The model under review builds one solid part; all positions refer to its coordinate system, in mm. A direction names the side the tool comes from. Coordinates: 2 decimals unless noted, no trailing zeros. Write each loop counter-clockwise with the first axis right and the second up, starting at its lowest first coordinate (ties: lowest second). Pieces come first, ordered by that corner, then holes. Notation, with made-up numbers: M 14,-9.5 L 37,-9.5 A12 ccw 37,2.5 Z; hole C 61,84 d2. An arc over 180 degrees is marked long. Answer as a JSON object with one key per item and string values.
Autodesk Fusion 360 part; units mm, degrees
sketch "Sketch1" plane through (0, 0, 0) normal (0, 0, 1) x (1, 0, 0)
  circle A0 centre (0, 0) radius 11
  circle A1 centre (0, 0) radius 12.5
  circle A2 centre (0, 0) radius 14.5
  line L0 (0, 0) -> (0, 14.5)
  line L1 (0, 0) -> (14.5, 0)
  line L2 (0, 0) -> (-14.5, 0)
  line L3 (0, 0) -> (0, -14.5)
  circle A3 centre (0, 14.5) radius 3.5
  circle A4 centre (14.5, 0) radius 3.5
  circle A5 centre (0, -14.5) radius 3.5
  circle A6 centre (-14.5, 0) radius 3.5
  circle A7 centre (-14.5, 0) radius 1.5
  circle A8 centre (0, 14.5) radius 1.5
  circle A9 centre (14.5, 0) radius 1.5
  circle A10 centre (0, -14.5) radius 1.5
  dimension "d1" = 22
  dimension "d2" = 25
  dimension "d3" = 29
  dimension "d4" = 7
  dimension "d5" = 3
  dimension "d6" = 3
  dimension "d7" = 3
  dimension "d8" = 3
extrude "Extrude1" add sketch "Sketch1" along normal blind 1 contours A0 A1 A4 A5 | A1 L1 A4 | A0 A1 A3 A4 | A1 L1 A4 | A1 L0 A3 | A0 A1 A3 A6 | A1 L0 A3 | A0 A1 A5 A6 | A1 L3 A5 | A1 L3 A5 | A1 A2 L1 A4 A9 | A1 A2 L1 A4 A9 | A1 A2 A3 A4 | A1 A2 A4 A5 | A1 L2 A6 | A1 L2 A6 | A1 A2 L0 A3 A8 | A1 A2 L0 A3 A8 | A1 A2 A3 A6 | A1 A2 L3 A5 A10 | A1 A2 L3 A5 A10 | A1 A2 A5 A6 | A2 A4 A9 | A1 A2 L2 A6 A7 | A1 A2 L2 A6 A7 | A2 A3 A8 | A2 A5 A10 | A2 A6 A7
sketch "Sketch2" plane through (0, 0, 1) normal (0, 0, 1) x (1, 0, 0)
  circle A0 centre (0, -14.5) radius 1.5
  circle A1 centre (14.5, 0) radius 1.5
  circle A2 centre (-14.5, 0) radius 1.5
  circle A3 centre (0, 14.5) radius 1.5
  circle A4 centre (0, 0) radius 11
  arc A5 (-3.4744, 14.0776) -> (-14.0776, 3.4744) centre (0, 0) ccw
  arc A6 (-14.0776, 3.4744) -> (-14.0776, -3.4744) centre (-14.5, 0) ccw
  arc A7 (-14.0776, -3.4744) -> (-3.4744, -14.0776) centre (0, 0) ccw
  arc A8 (-3.4744, -14.0776) -> (3.4744, -14.0776) centre (0, -14.5) ccw
  arc A9 (3.4744, -14.0776) -> (14.0776, -3.4744) centre (0, 0) ccw
  arc A10 (14.0776, -3.4744) -> (14.0776, 3.4744) centre (14.5, 0) ccw
  arc A11 (14.0776, 3.4744) -> (3.4744, 14.0776) centre (0, 0) ccw
  arc A12 (3.4744, 14.0776) -> (-3.4744, 14.0776) centre (0, 14.5) ccw
  circle A13 centre (0, 0) radius 11
  circle A14 centre (0, 0) radius 12.375
  circle A15 centre (0, 0) radius 14.5
  circle A16 centre (0, 14.5) radius 3.5
  circle A17 centre (14.5, 0) radius 3.5
  circle A18 centre (0, -14.5) radius 3.5
  circle A19 centre (-14.5, 0) radius 3.5
  dimension "d11" = 24.75
extrude "Extrude2" add sketch "Sketch2" along normal blind 1.25 contours A0 A8 A15 A18 | A0 A14 A15 A18 | A9 A14 A15 A17 A18 | A7 A14 A15 A18 A19 | A1 A10 A15 A17 | A1 A14 A15 A17 | A2 A6 A15 A19 | A2 A14 A15 A19 | A5 A14 A15 A16 A19 | A11 A14 A15 A16 A17 | A3 A12 A15 A16 | A3 A14 A15 A16
extrude "Extrude3" cut 1 faces at (-2.5265, -13.3305, 2.25) along direction (0, 0, -1) blind 1.25
sketch "Sketch3" plane through (0, 0, 1) normal (0, 0, 1) x (1, 0, 0)
  arc A0 (-3.4744, 14.0776) -> (-14.0776, 3.4744) centre (0, 0) ccw
  arc A1 (-14.0776, 3.4744) -> (-14.0776, -3.4744) centre (-14.5, 0) ccw
  arc A2 (-14.0776, -3.4744) -> (-3.4744, -14.0776) centre (0, 0) ccw
  arc A3 (-3.4744, -14.0776) -> (3.4744, -14.0776) centre (0, -14.5) ccw
  arc A4 (3.4744, -14.0776) -> (14.0776, -3.4744) centre (0, 0) ccw
  arc A5 (14.0776, -3.4744) -> (14.0776, 3.4744) centre (14.5, 0) ccw
  arc A6 (14.0776, 3.4744) -> (3.4744, 14.0776) centre (0, 0) ccw
  arc A7 (3.4744, 14.0776) -> (-3.4744, 14.0776) centre (0, 14.5) ccw
  circle A8 centre (0, 14.5) radius 1.5
  circle A9 centre (14.5, 0) radius 1.5
  circle A10 centre (-14.5, 0) radius 1.5
  circle A11 centre (0, -14.5) radius 1.5
  circle A12 centre (0, 0) radius 11
  circle A13 centre (0, 0) radius 3.05
  dimension "d16" = 6.1
extrude "Extrude4" add sketch "Sketch3" along normal blind 2 contours A0 A1 A2 A3 A4 A5 A6 A7 | A12
sketch "Sketch4" plane through (0, 0, 3) normal (0, 0, 1) x (1, 0, 0)
  circle A0 centre (-14.5, 0) radius 1.5
  circle A1 centre (0, 14.5) radius 1.5
  circle A2 centre (0, 0) radius 3.05
  circle A3 centre (0, -14.5) radius 1.5
  circle A4 centre (14.5, 0) radius 1.5
  arc A5 (3.4744, 14.0776) -> (-3.4744, 14.0776) centre (0, 14.5) ccw
  arc A6 (-3.4744, 14.0776) -> (-14.0776, 3.4744) centre (0, 0) ccw
  arc A7 (-14.0776, 3.4744) -> (-14.0776, -3.4744) centre (-14.5, 0) ccw
  arc A8 (-14.0776, -3.4744) -> (-3.4744, -14.0776) centre (0, 0) ccw
  arc A9 (-3.4744, -14.0776) -> (3.4744, -14.0776) centre (0, -14.5) ccw
  arc A10 (3.4744, -14.0776) -> (14.0776, -3.4744) centre (0, 0) ccw
  arc A11 (14.0776, -3.4744) -> (14.0776, 3.4744) centre (14.5, 0) ccw
  arc A12 (14.0776, 3.4744) -> (3.4744, 14.0776) centre (0, 0) ccw
  circle A13 centre (0, 0) radius 1.5
  dimension "d19" = 3
extrude "Extrude5" cut sketch "Sketch4" against normal blind 1 contours A5 A6 A7 A8 A9 A10 A11 A12
sketch "Sketch5" plane through (0, 0, 2) normal (0, 0, 1) x (1, 0, 0)
  circle A0 centre (0, -14.5) radius 1.5
  circle A1 centre (0, 0) radius 3.05
  circle A2 centre (14.5, 0) radius 1.5
  circle A3 centre (0, 14.5) radius 1.5
  circle A4 centre (-14.5, 0) radius 1.5
  arc A5 (14.0776, 3.4744) -> (3.4744, 14.0776) centre (0, 0) ccw
  arc A6 (3.4744, 14.0776) -> (-3.4744, 14.0776) centre (0, 14.5) ccw
  arc A7 (-3.4744, 14.0776) -> (-14.0776, 3.4744) centre (0, 0) ccw
  arc A8 (-14.0776, 3.4744) -> (-14.0776, -3.4744) centre (-14.5, 0) ccw
  arc A9 (-14.0776, -3.4744) -> (-3.4744, -14.0776) centre (0, 0) ccw
  arc A10 (-3.4744, -14.0776) -> (3.4744, -14.0776) centre (0, -14.5) ccw
  arc A11 (3.4744, -14.0776) -> (14.0776, -3.4744) centre (0, 0) ccw
  arc A12 (14.0776, -3.4744) -> (14.0776, 3.4744) centre (14.5, 0) ccw
  circle A13 centre (0, 0) radius 3.05
  circle A14 centre (0, 0) radius 4
  dimension "d22" = 8
extrude "Extrude6" add sketch "Sketch5" along normal blind 4 contours A14
chamfer "Chamfer1" distance 2 angle 45 1 edges at (-3.7293, 1.4465, 2)
extrude "Extrude7" add 1 faces at (8.2977, -0.698, 1) along direction (0, 0, -1) blind 1
sketch "Sketch7" plane through (0, 0, 6) normal (0, 0, 1) x (1, 0, 0)
  circle A0 centre (0, 0) radius 3.05
  circle A1 centre (0, 0) radius 4
  circle A2 centre (0, 0) radius 3.125
  dimension "d28" = 6.25
extrude "Extrude8" cut sketch "Sketch7" against normal blind 100 contours A2
(1) Wall thickness on line 1 along Y through (x, z) = (0, 1.4) (3 decimals); line 2 along Y through (x, z) = (-14.5, 0.9); line 3 along Y through (x, z) = (0, 4.65) (3 decimals): over which ranges is each line inside the solid? List them lowest first. Write a range as from..to.
Results list:
{"line 1": "-18..-16, -13..-3.125, 3.125..13, 16..18", "line 2": "-3.5..-1.5, 1.5..3.5", "line 3": "-4..-3.125, 3.125..4"}
(2) For faces 4 (the face through (-0.867, 3.905, 4.986)), 5 (the face through (2, -3, 6)), list the 3-axis set-ups (+Z, -Z, +X, -X, +Y, -Y) from which the entire face can be reached by the end or side of a thin tool; tool diameter is ignored.
Results list:
{"face 4": "+Z", "face 5": "+Z, +X, -X, +Y, -Y"}
(3) Add section C-C on y = -15.5. Give the boundary of the cut face in (x, z).
Results list:
{"outline": "M -3.35,0 L -1.12,0 L -1.12,2 L -3.35,2 Z; M 1.12,0 L 3.35,0 L 3.35,2 L 1.12,2 Z"}
(4) For pin 1 Ø1.5 at (y, z) = (-2.5, 2) entering from +X, flat-tipped, find the tip position at first contact; note if it passes through.
Results list:
{"pin 1": "x = 17.53"}
(5) Add section A-A on y = 0. Give the boundary of the cut face in (x, z) (3 decimals).
Results list:
{"outline": "M -18,0 L -16,0 L -16,2 L -18,2 Z; M -13,0 L -3.125,0 L -3.125,6 L -4,6 L -4,4 L -6,2 L -13,2 Z; M 3.125,0 L 13,0 L 13,2 L 6,2 L 4,4 L 4,6 L 3.125,6 Z; M 16,0 L 18,0 L 18,2 L 16,2 Z"}
(6) Add section D-D on x = 14.5. Give the boundary of the cut face in (y, z), and give its area (3 significant figures).
Results list:
{"outline": "M -3.5,0 L -1.5,0 L -1.5,2 L -3.5,2 Z; M 1.5,0 L 3.5,0 L 3.5,2 L 1.5,2 Z", "area": "8.00 mm²"}
(7) Draft analysis for pull direction Y (two halves, no side actions). For faces 1 (the face through (18, 0.1, 0.5)), 2 (the face through (0, -13, 1)), 3 (the face through (8, 0, 2)), state which applies: released by +Y, released by -Y, zero draft, split by the parting line, or undercut.
Results list:
{"face 1": "split by the parting line", "face 2": "undercut", "face 3": "zero draft"}
